from build123d import *

# Parameters (mm, degrees)
BOSS_EXTRUDE1_DEPTH = 0.8
BOSS_EXTRUDE2_DEPTH = 9.525
FILLET1_R           = 1.27


with BuildPart() as part:
    # Sketch1 → Boss-Extrude1 (new body)
    with BuildSketch(Plane.XY):
        Polygon((0, 0), (0, 15.697000102), (6.172000102, 15.697000102), (6.172000102, 6.172000102), (15.697000102, 6.172000102), (15.697000102, 0), align=None)
    extrude(amount=BOSS_EXTRUDE1_DEPTH)

    # Sketch2 → Boss-Extrude2 (add)
    with BuildSketch(Plane.XY.offset(0.8)):
        Polygon((0.8, 0.8), (15.697000102, 0.8), (15.697000102, 0), (0, 0), (0, 15.697000102), (0.8, 15.697000102), align=None)
        Polygon((15.697000102, 5.372000102), (5.372000102, 5.372000102), (5.372000102, 15.697000102), (6.172000102, 15.697000102), (6.172000102, 6.172000102), (15.697000102, 6.172000102), align=None)
    extrude(amount=BOSS_EXTRUDE2_DEPTH)

    # Fillet1
    fillet1_edges = [part.edges().sort_by_distance(p)[0] for p in [
        (6.172000102, 6.172000102, 5.1625),
        (5.372000102, 5.372000102, 5.5625),
    ]]
    fillet(fillet1_edges, radius=FILLET1_R)


solid = part.part
For this review, take the finished solid that the model builds, in its own axes (mm). A direction names the side the tool comes from. Coordinates: 2 decimals unless noted, no trailing zeros. Order: outer loops, then holes, each group sorted by start corner. A loop starts at its lowest first (then second) coordinate and runs counter-clockwise, first axis right, second up. Notation, with made-up numbers: (21, -3.75) -> (61, -3.75) arc R34 ccw to (61, 29.25) -> close; hole circle Ø3 at (-14.75, -32.75). An arc over 180 degrees is marked (long way). Return JSON: item names as keys, results as strings.
1. We need section A-A on z = 1.25. Write out the cut boundary in (x, y).
Answer block:
{"outline": "(0, 0) -> (15.7, 0) -> (15.7, 0.8) -> (0.8, 0.8) -> (0.8, 15.7) -> (0, 15.7) -> close; (5.37, 6.64) arc R1.27 ccw to (6.64, 5.37) -> (15.7, 5.37) -> (15.7, 6.17) -> (7.44, 6.17) arc R1.27 cw to (6.17, 7.44) -> (6.17, 15.7) -> (5.37, 15.7) -> close"}
2. We need section B-B on y = 9. Write out the cut boundary in (x, z) (3 decimals), and give its area (3 significant figures).
Answer block:
{"outline": "(0, 0) -> (6.172, 0) -> (6.172, 10.325) -> (5.372, 10.325) -> (5.372, 0.8) -> (0.8, 0.8) -> (0.8, 10.325) -> (0, 10.325) -> close", "area": "20.2 mm²"}
3. The part is to be moulded in two halves that separate along Y. For faces 1 (the flat face through (5.372, 11, 5)), 2 (the flat face through (8, 0.8, 5)), 3 (the cylindrical face through (6.554, 6.534, 5.235)), 4 (the flat face through (8, 0, 5)), say which applies: +Y half, -Y half, draft (parallel to the pull), parting line (faces both ways), or undercut.
Answer block:
{"face 1": "draft", "face 2": "undercut", "face 3": "+Y half", "face 4": "-Y half"}
4. We need section C-C on x = 4.25. Write out the cut boundary in (y, z) (3 decimals).
Answer block:
{"outline": "(0, 0) -> (15.697, 0) -> (15.697, 0.8) -> (0.8, 0.8) -> (0.8, 10.325) -> (0, 10.325) -> close"}
5. Machinability: for faces 5 (the flat face through (5, 7, 0.8)), 6 (the flat face through (0.8, 8, 5)), 7 (the flat face through (6.172, 12, 5)), which of the approach directions +Z, -Z, +X, -X, +Y, -Y give a long, thin tool a straight path to every point of the face, cutting with its end or side? Answer none if there is none.
Answer block:
{"face 5": "+Z", "face 6": "+Z, +Y", "face 7": "+Z, -Z, +X, +Y"}
6. For line 1 (X direction, y = 13, z = 8.75); line 2 (Z direction, x = 3.5, y = 13.5), list the stretches that pass through material, from the lowest coordinate up. Write a range as from..to.
Answer block:
{"line 1": "0..0.8, 5.37..6.17", "line 2": "0..0.8"}
7. For pin 1 Ø8 at (x, y) = (10.5, 11.5) entering from +Z; pin 2 Ø1.5 at (y, z) = (3.5, 8) entering from +X; pin 3 Ø1 at (y, z) = (12, 8.5) entering from +X; pin 4 Ø1.5 at (x, z) = (7.5, 6.5) entering from +Y, all flat-tipped, find the tip position at first contact; note any pin that passes through.
Answer block:
{"pin 1": "through", "pin 2": "x = 0.8", "pin 3": "x = 6.17", "pin 4": "y = 6.38"}
